```python
from build123d import *

# Parameters (mm, degrees)
SKETCH_1_W          = 85
SKETCH_1_H          = 45
EXTRUDE_1_DEPTH     = 125
SKETCH_2_W          = 81.8
SKETCH_2_H          = 41.8
CUT_EXTRUDE_1_DEPTH = 123.4
SKETCH_3_W          = 83.4
SKETCH_3_H          = 43.4
CUT_EXTRUDE_2_DEPTH = 4
FILLET_2_R          = 1


with BuildPart() as part:
    # Эскиз1 → Бобышка-Вытянуть1 (new body)
    with BuildSketch(Plane.XY):
        with Locations((42.5, 22.5)):
            Rectangle(SKETCH_1_W, SKETCH_1_H)
    extrude(amount=EXTRUDE_1_DEPTH)

    # Эскиз2 → Вырез-Вытянуть1 (cut)
    with BuildSketch(Plane.XY.offset(125)):
        with Locations((42.5, 22.5)):
            Rectangle(SKETCH_2_W, SKETCH_2_H)
    extrude(amount=-CUT_EXTRUDE_1_DEPTH, mode=Mode.SUBTRACT)

    # Эскиз3 → Вырез-Вытянуть2 (cut)
    with BuildSketch(Plane.XY.offset(125)):
        with Locations((42.5, 22.5)):
            Rectangle(SKETCH_3_W, SKETCH_3_H)
    extrude(amount=-CUT_EXTRUDE_2_DEPTH, mode=Mode.SUBTRACT)

    # Скругление2
    fillet_2_edges = [part.edges().sort_by_distance(p)[0] for p in [
        (0, 45, 62.5),
        (85, 45, 62.5),
        (85, 0, 62.5),
        (0, 0, 62.5),
    ]]
    fillet(fillet_2_edges, radius=FILLET_2_R)


solid = part.part
```
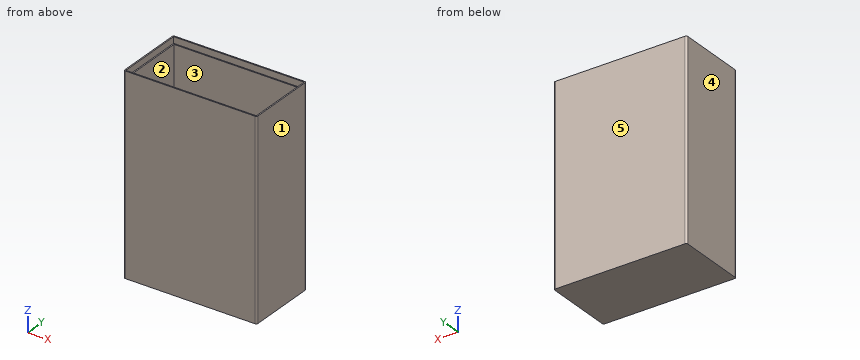
CAD build for the part. Positions are in the model's coordinates, mm. Face numbers are marked on the shaded views. A direction names the side the tool comes from. Round coordinates to 2 decimals unless told otherwise and drop trailing zeros. Loops run counter-clockwise (first coordinate to the right, second up) from the corner with the lowest first, then second, coordinate; pieces in that order, holes last. Notation, with made-up numbers: (80, 54) - (122, 54) arc R25 ccw to (122, 81) - close; hole circle Ø11 at (-11, 13.25). An arc over 180 degrees is marked (long way). Return JSON: item names as keys, results as strings. Group by question number.
Q1. Drill centre lines: line 1 along X through (y, z) = (41, 105); line 2 along Y through (x, z) = (5.5, 47); line 3 along Z through (x, y) = (81, 37). Where is each one in solid material? Low to high. Write a range as [from, to].
Q2. Band-saw the part on B-B on x = 41.5. Give the cut face in (y, z).
Q3. Flat gauge pins, fed straight in: pin 1 Ø1 at (x, y) = (61, 22) entering from -Z; pin 2 Ø12.5 at (x, y) = (28, 27.5) entering from +Z. Where does each tip first touch, or does it go through?
Q4. Two-plate mould, pull along Y, no slides. Class the marked faces 3, 4 and 5: +Y half, -Y half, draft (parallel to the pull), parting line (faces both ways), or undercut.
Q5. Tool access for the marked faces 1 and 2: list every direction of +Z, -Z, +X, -X, +Y, -Y with a clear straight run to the whole face (end or side of a thin tool).
Q6. Band-saw the part on A-A on z = 78. Give the cut face in (x, y).
Q7. Band-saw the part on C-C on y = 4.5. Give the cut face in (x, z), plus the area to 3 significant figures.
Solutions:
{
 "1": {"line 1": "x = [0, 1.6], [83.4, 85]", "line 2": "y = [0, 1.6], [43.4, 45]", "line 3": "z = [0, 1.6]"},
 "2": {"outline": "(0, 0) - (45, 0) - (45, 125) - (44.2, 125) - (44.2, 121) - (43.4, 121) - (43.4, 1.6) - (1.6, 1.6) - (1.6, 121) - (0.8, 121) - (0.8, 125) - (0, 125) - close"},
 "3": {"pin 1": "stops at z = 0", "pin 2": "stops at z = 1.6"},
 "4": {"face 3": "undercut", "face 4": "draft", "face 5": "+Y half"},
 "5": {"face 1": "+Z, -Z, +X, +Y, -Y", "face 2": "+Z"},
 "6": {"outline": "(0, 1) arc R1 ccw to (1, 0) - (84, 0) arc R1 ccw to (85, 1) - (85, 44) arc R1 ccw to (84, 45) - (1, 45) arc R1 ccw to (0, 44) - close; hole (1.6, 1.6) - (83.4, 1.6) - (83.4, 43.4) - (1.6, 43.4) - close"},
 "7": {"outline": "(0, 0) - (85, 0) - (85, 125) - (84.2, 125) - (84.2, 121) - (83.4, 121) - (83.4, 1.6) - (1.6, 1.6) - (1.6, 121) - (0.8, 121) - (0.8, 125) - (0, 125) - close", "area": "524 mm^2"}
}
